Part model, mm, in its own coordinate system. Face numbers are marked on the shaded views. Give positions to 0.01 mm unless a question says otherwise; leave off trailing zeros. Write each loop counter-clockwise with the first axis right and the second up, starting at its lowest first coordinate (ties: lowest second). Pieces come first, ordered by that corner, then holes. Notation, with made-up numbers: (-32, -36) - (-25, -36) arc R31 ccw to (-25, -3) - close; hole circle Ø10 at (62, 75.25). An arc over 180 degrees is marked (long way). Answer as a JSON object with one key per item and string values. Group by question number.
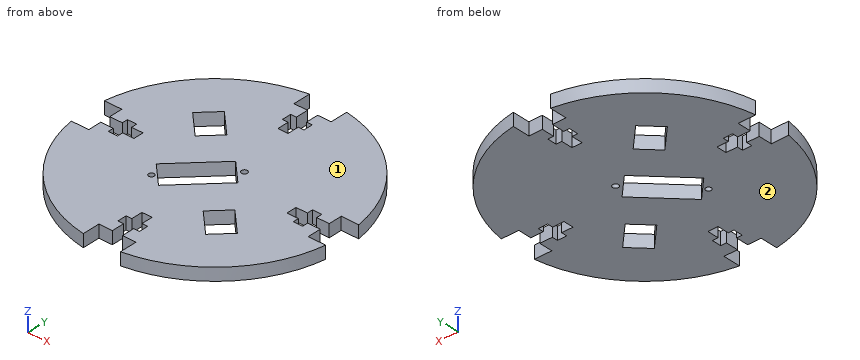
```python
from build123d import *

# Parameters (mm, degrees)
SKETCH3_R           = 1.089052178
SKETCH3_R_2         = 1.175054292
BOSS_EXTRUDE5_DEPTH = 5


with BuildPart() as part:
    # Sketch3 → Boss-Extrude5 (new body)
    with BuildSketch(Plane.XY):
        with BuildLine():
            Line((81.038403504, 109.892462561), (81.038403504, 102.992462561))
            Line((81.038403504, 102.992462561), (75.701022894, 102.992462561))
            Line((75.701022894, 102.992462561), (75.701022894, 98.038427684))
            Line((75.701022894, 98.038427684), (77.959022894, 98.038427684))
            Line((77.959022894, 98.038427684), (77.959022894, 94.370627684))
            Line((77.959022894, 94.370627684), (75.701022894, 94.370627684))
            Line((75.701022894, 94.370627684), (75.701022894, 89.854027684))
            Line((75.701022894, 89.854027684), (71.701022894, 89.854027684))
            Line((71.701022894, 89.854027684), (71.701022894, 94.370627684))
            Line((71.701022894, 94.370627684), (69.443022894, 94.370627684))
            Line((69.443022894, 94.370627684), (69.443022894, 98.038427684))
            Line((69.443022894, 98.038427684), (71.701022894, 98.038427684))
            Line((71.701022894, 98.038427684), (71.701022894, 102.992462561))
            Line((71.701022894, 102.992462561), (66.363642284, 102.992462561))
            Line((66.363642284, 102.992462561), (66.363642284, 109.892462561))
            ThreePointArc((66.363642284, 109.892462561), (37.802245989, 95.555722027), (23.465505456, 66.994325733))
            Line((23.465505456, 66.994325733), (30.365505456, 66.994325733))
            Line((30.365505456, 66.994325733), (30.365505456, 61.656945123))
            Line((30.365505456, 61.656945123), (35.319540332, 61.656945123))
            Line((35.319540332, 61.656945123), (35.319540332, 63.914945123))
            Line((35.319540332, 63.914945123), (38.987340332, 63.914945123))
            Line((38.987340332, 63.914945123), (38.987340332, 61.656945123))
            Line((38.987340332, 61.656945123), (43.503940332, 61.656945123))
            Line((43.503940332, 61.656945123), (43.503940332, 57.656945123))
            Line((43.503940332, 57.656945123), (38.987340332, 57.656945123))
            Line((38.987340332, 57.656945123), (38.987340332, 55.398945123))
            Line((38.987340332, 55.398945123), (35.319540332, 55.398945123))
            Line((35.319540332, 55.398945123), (35.319540332, 57.656945123))
            Line((35.319540332, 57.656945123), (30.365505456, 57.656945123))
            Line((30.365505456, 57.656945123), (30.365505456, 52.319564513))
            Line((30.365505456, 52.319564513), (23.465505456, 52.319564513))
            ThreePointArc((23.465505456, 52.319564513), (37.802245989, 23.758168218), (66.363642284, 9.421427684))
            Line((66.363642284, 9.421427684), (66.363642284, 16.321427684))
            Line((66.363642284, 16.321427684), (71.701022894, 16.321427684))
            Line((71.701022894, 16.321427684), (71.701022894, 21.275462561))
            Line((71.701022894, 21.275462561), (69.443022894, 21.275462561))
            Line((69.443022894, 21.275462561), (69.443022894, 24.943262561))
            Line((69.443022894, 24.943262561), (71.701022894, 24.943262561))
            Line((71.701022894, 24.943262561), (71.701022894, 29.459862561))
            Line((71.701022894, 29.459862561), (75.701022894, 29.459862561))
            Line((75.701022894, 29.459862561), (75.701022894, 24.943262561))
            Line((75.701022894, 24.943262561), (77.959022894, 24.943262561))
            Line((77.959022894, 24.943262561), (77.959022894, 21.275462561))
            Line((77.959022894, 21.275462561), (75.701022894, 21.275462561))
            Line((75.701022894, 21.275462561), (75.701022894, 16.321427684))
            Line((75.701022894, 16.321427684), (81.038403504, 16.321427684))
            Line((81.038403504, 16.321427684), (81.038403504, 9.421427684))
            ThreePointArc((81.038403504, 9.421427684), (109.599799799, 23.758168218), (123.936540332, 52.319564513))
            Line((123.936540332, 52.319564513), (117.036540332, 52.319564513))
            Line((117.036540332, 52.319564513), (117.036540332, 57.656945123))
            Line((117.036540332, 57.656945123), (112.082505456, 57.656945123))
            Line((112.082505456, 57.656945123), (112.082505456, 55.398945123))
            Line((112.082505456, 55.398945123), (108.414705456, 55.398945123))
            Line((108.414705456, 55.398945123), (108.414705456, 57.656945123))
            Line((108.414705456, 57.656945123), (103.898105456, 57.656945123))
            Line((103.898105456, 57.656945123), (103.898105456, 61.656945123))
            Line((103.898105456, 61.656945123), (108.414705456, 61.656945123))
            Line((108.414705456, 61.656945123), (108.414705456, 63.914945123))
            Line((108.414705456, 63.914945123), (112.082505456, 63.914945123))
            Line((112.082505456, 63.914945123), (112.082505456, 61.656945123))
            Line((112.082505456, 61.656945123), (117.036540332, 61.656945123))
            Line((117.036540332, 61.656945123), (117.036540332, 66.994325733))
            Line((117.036540332, 66.994325733), (123.936540332, 66.994325733))
            ThreePointArc((123.936540332, 66.994325733), (109.599799799, 95.555722027), (81.038403504, 109.892462561))
        make_face()
        with Locations((60.382249582, 46.393077684)):
            Circle(SKETCH3_R, mode=Mode.SUBTRACT)
        Polygon((65.663040298, 43.594110186), (57.487806829, 51.769189843), (74.099869727, 68.381565292), (82.275103197, 60.206485634), align=None, mode=Mode.SUBTRACT)
        Polygon((93.597305456, 33.128564513), (84.692315031, 42.034629122), (91.325115031, 48.666629122), (100.230105456, 39.760564513), align=None, mode=Mode.SUBTRACT)
        Polygon((56.078706893, 70.64823726), (47.172642284, 79.553227684), (53.804642284, 86.186027684), (62.710706893, 77.28103726), align=None, mode=Mode.SUBTRACT)
        with Locations((79.827503135, 65.838697094)):
            Circle(SKETCH3_R_2, mode=Mode.SUBTRACT)
    extrude(amount=BOSS_EXTRUDE5_DEPTH)


solid = part.part
```
1) Band-saw the part on B-B (x = 32.5). List the corners of the cut face in (y, z), plus the area to 3 significant figures.
2) Probe line 1 (Y direction, x = 62, z = 0.4); line 2 (X direction, y = 45.5, z = 1.25); line 3 (X direction, y = 57, z = 3.6). List the from-to ranges inside material, lowest first.
3) Mould opens along Z. For the marked faces 1 and 2 say: pulls with the +Z half, pulls with the -Z half, needs draft (parallel to the pull), parting line crosses it, or undercut.
4) Drop flat-ended pins along their axis: P1, Ø0.7, axis at x = 71, z = 1.5, coming from the -Y side; P2, Ø1.5, axis at x = 49, z = 3, coming from the -Y side; P3, Ø1.5, axis at y = 21, z = 3, coming from the -X side. Give the stop position or say it passes through.
5) Band-saw the part on A-A (x = 95.5). List the corners of the cut face in (y, z), plus the area to 3 significant figures.
6) Band-saw the part on C-C (z = 3.25). State how many separate pieces and enclosed holes the cut face has, plus the area to 3 significant figures.
Verdict:
{
 "1": {"outline": "(29.99, 0) - (57.66, 0) - (57.66, 5) - (29.99, 5) - close; (61.66, 0) - (89.32, 0) - (89.32, 5) - (61.66, 5) - close", "area": "277 mm2"},
 "2": {"line 1": "10.26 to 47.26, 56.28 to 76.57, 77.99 to 109.06", "line 2": "24.95 to 59.76, 61.01 to 63.76, 67.57 to 88.16, 94.49 to 122.46", "line 3": "30.37 to 35.32, 38.99 to 62.72, 79.07 to 108.41, 112.08 to 117.04"},
 "3": {"face 1": "pulls with the +Z half", "face 2": "pulls with the -Z half"},
 "4": {"P1": "y = 16.32", "P2": "y = 14.89", "P3": "x = 39.93"},
 "5": {"outline": "(13.81, 0) - (35.03, 0) - (35.03, 5) - (13.81, 5) - close; (44.49, 0) - (105.51, 0) - (105.51, 5) - (44.49, 5) - close", "area": "411 mm2"},
 "6": {"separate pieces": "1", "enclosed holes": "5", "area": "6,880 mm2"}
}
